Here's how the part is built. I have some questions about the finished solid (model axes, mm). Face numbers are marked on the shaded views. A direction names the side the tool comes from. Give positions to 0.01 mm unless a question says otherwise; leave off trailing zeros. Write each loop counter-clockwise with the first axis right and the second up, starting at its lowest first coordinate (ties: lowest second). Pieces come first, ordered by that corner, then holes. Notation, with made-up numbers: (64, -26) - (80, -26) arc R35 cw to (80, 6) - close; hole circle Ø10 at (6.25, 74.25). An arc over 180 degrees is marked (long way). One line per item, written item: value. Start each with the question number.
1) Imagine slicing it at C-C on x = -51.5. Write out the boundary of the cut face in (y, z) (3 decimals).
2) Imagine slicing it at B-B on y = 42. Write out the boundary of the cut face in (x, z) (3 decimals), plus the area to 3 significant figures.
3) I'm going to push flat-ended pins straight in: P1, Ø7.5, axis at y = -6, z = -5.5, coming from the -X side; P2, Ø4.5, axis at y = 8.5, z = 0, coming from the -X side; P3, Ø7, axis at x = 1, z = 7.5, coming from the +Y side; P4, Ø3.5, axis at x = -46.88, y = 72.87, coming from the -Z side. Where does each tip first touch, or does it pass through?
4) Imagine slicing it at A-A on z = 8.5. Write out the boundary of the cut face in (x, y) (3 decimals).
5) We'd pull the mould along Z, two halves only. Please class the marked faces 1, 2 and 3: +Z half, -Z half, draft (parallel to the pull), parting line (faces both ways), or undercut.
6) Imagine slicing it at D-D on y = 0. Count the separate pieces of the cut face and the enclosed holes in it, plus the area to 3 significant figures.
7) Please list where these lines run through material, in increasing order: L1, parallel to Y at x = 2.75, z = 0; L2, parallel to Z at x = 2, y = 0; L3, parallel to Z at x = -31, y = 48 (3 decimals). Write a range as [from, to].
8) On a 3-axis mill with a long thin cutter (end or side, diameter ignored), from which of +Z, -Z, +X, -X, +Y, -Y can I reach the whole of each face in a straight line? I mean the marked faces 4 and 5. Say none if no direction works.
from build123d import *

# Parameters (mm, degrees)
SKETCH2_W                                      = 29
SKETCH2_H                                      = 25
BOSS_EXTRUDE1_DEPTH                            = 6.35
CONVERT_SOLID1_START                           = 3.175
CONVERT_SOLID1_OUTLINE_W                       = 25
CONVERT_SOLID1_OUTLINE_H                       = 29
CONVERT_SOLID1_DEPTH                           = 3.175
CSK_FOR_M3_5_FLAT_HEAD_MACHINE_SCREW1_AT_COUNT = 2
CSK_FOR_M3_5_FLAT_HEAD_MACHINE_SCREW1_AT_PITCH = 12.02081528
CSK_FOR_M3_5_FLAT_HEAD_MACHINE_SCREW_2_COUNT   = 2
CSK_FOR_M3_5_FLAT_HEAD_MACHINE_SCREW_2_PITCH   = 17
CSK_FOR_M3_5_FLAT_HEAD_MACHINE_SCREW_3_COUNT   = 2
CSK_FOR_M3_5_FLAT_HEAD_MACHINE_SCREW_3_PITCH   = 12.02081528
EDGE_FLANGE1_DEPTH                             = 25
EDGE_FLANGE1_BEND_DEPTH                        = 25
SKETCH23_R                                     = 1.95
SKETCH23_R_2                                   = 6.875
BOSS_EXTRUDE2_DEPTH                            = 3.175
FILLET1_R                                      = 40
SKETCH25_R                                     = 1.95
SKETCH25_R_2                                   = 6.875
CUT_EXTRUDE3_DEPTH                             = 108.532674661
FILLET2_R                                      = 2


# Read off the part's stored shape, not the designer's step: Convert-Solid1
# Sheet-metal steps are written as plain solids
with BuildPart() as part:
    # Sketch2 → Boss-Extrude1 (new body)
    with BuildSketch(Plane(origin=(0, 0, 0), x_dir=(0, 0, -1), z_dir=(1, 0, 0))):
        Rectangle(SKETCH2_W, SKETCH2_H)
    extrude(amount=BOSS_EXTRUDE1_DEPTH)

    # Convert-Solid1 outline → Convert-Solid1 (cut)
    with BuildSketch(Plane.YZ.offset(CONVERT_SOLID1_START)):
        Rectangle(CONVERT_SOLID1_OUTLINE_W, CONVERT_SOLID1_OUTLINE_H)
    extrude(amount=CONVERT_SOLID1_DEPTH, mode=Mode.SUBTRACT)

    # Sketch4 → CSK for M3.5 Flat Head Machine Screw1 (revolve, cut)
    with BuildSketch(Plane.ZX.offset(-8.5)):
        Polygon((0, 0), (0, 3.175), (1.95, 3.175), (1.95, 2.15), (4.1, 0), align=None)
    csk_for_m3_5_flat_head_machine_screw1 = revolve(axis=Axis((-6.35, -8.5, 0), (1, 0, 0)), mode=Mode.SUBTRACT)

    # CSK for M3.5 Flat Head Machine Screw1 at: CSK for M3.5 Flat Head Machine Screw1 ×2
    with Locations(*[Vector(0, 0.7071067811865476, 0.7071067811865476) * (i * CSK_FOR_M3_5_FLAT_HEAD_MACHINE_SCREW1_AT_PITCH) for i in range(1, CSK_FOR_M3_5_FLAT_HEAD_MACHINE_SCREW1_AT_COUNT)]):
        add(csk_for_m3_5_flat_head_machine_screw1, mode=Mode.SUBTRACT)

    # CSK for M3.5 Flat Head Machine Screw 2: CSK for M3.5 Flat Head Machine Screw1 ×2
    with Locations(*[(0, i * CSK_FOR_M3_5_FLAT_HEAD_MACHINE_SCREW_2_PITCH, 0) for i in range(1, CSK_FOR_M3_5_FLAT_HEAD_MACHINE_SCREW_2_COUNT)]):
        add(csk_for_m3_5_flat_head_machine_screw1, mode=Mode.SUBTRACT)

    # CSK for M3.5 Flat Head Machine Screw 3: CSK for M3.5 Flat Head Machine Screw1 ×2
    with Locations(*[Vector(0, 0.7071067811865476, -0.7071067811865476) * (i * CSK_FOR_M3_5_FLAT_HEAD_MACHINE_SCREW_3_PITCH) for i in range(1, CSK_FOR_M3_5_FLAT_HEAD_MACHINE_SCREW_3_COUNT)]):
        add(csk_for_m3_5_flat_head_machine_screw1, mode=Mode.SUBTRACT)

    # Edge-Flange1 section (across the edge) → Edge-Flange1 (add)
    with BuildSketch(Plane(origin=(0, 12.5, -17.675), x_dir=(0, 0, 1), z_dir=(0, -1, 0))):
        with BuildLine():
            Line((-3.175, 3.175), (-3.175, 36.825))
            Line((-3.175, 36.825), (0, 36.825))
            Line((0, 36.825), (0, 3.175))
            ThreePointArc((0, 3.175), (0.92993597, 0.92993597), (3.175, 0))
            Line((3.175, 0), (3.175, -3.175))
            ThreePointArc((3.175, -3.175), (-1.315128061, -1.315128061), (-3.175, 3.175))
        make_face()
    extrude(amount=EDGE_FLANGE1_DEPTH)

    # Edge-Flange1 section 2 (across the edge) → Edge-Flange1 bend (add)
    with BuildSketch(Plane(origin=(0, -12.5, 17.675), x_dir=(0, 0, -1), z_dir=(0, 1, 0))):
        with BuildLine():
            Line((-3.175, 3.175), (-3.175, 36.825))
            Line((-3.175, 36.825), (0, 36.825))
            Line((0, 36.825), (0, 3.175))
            ThreePointArc((0, 3.175), (0.92993597, 0.92993597), (3.175, 0))
            Line((3.175, 0), (3.175, -3.175))
            ThreePointArc((3.175, -3.175), (-1.315128061, -1.315128061), (-3.175, 3.175))
        make_face()
    extrude(amount=EDGE_FLANGE1_BEND_DEPTH)

    # Sketch23 → Boss-Extrude2 (add)
    with BuildSketch(Plane.XY.offset(20.85)):
        with BuildLine():
            Line((-3.175, -12.5), (-3.175, 12.5))
            Line((-3.175, 12.5), (-39.000765285, 77.226355048))
            ThreePointArc((-39.000765285, 77.226355048), (-50.077531286, 81.278922457), (-55.654025191, 70.885618681))
            Line((-55.654025191, 70.885618681), (-36.825, -12.5))
            Line((-36.825, -12.5), (-3.175, -12.5))
        make_face()
        with Locations((-46.875056501, 72.867967978)):
            Circle(SKETCH23_R, mode=Mode.SUBTRACT)
        with Locations((-29.474943499, 27.168448642)):
            Circle(SKETCH23_R, mode=Mode.SUBTRACT)
        with Locations((-38.175, 50.01820831)):
            Circle(SKETCH23_R_2, mode=Mode.SUBTRACT)
    boss_extrude2 = extrude(amount=-BOSS_EXTRUDE2_DEPTH)

    # Mirror3: Boss-Extrude2 across plane
    add(boss_extrude2.mirror(Plane.XY))

    # Fillet1
    fillet1_edges = [part.edges().sort_by_distance(p)[0] for p in [
        (-36.825, -12.5, -19.2625),
        (-36.825, -12.5, 19.2625),
    ]]
    fillet(fillet1_edges, radius=FILLET1_R)

    # Sketch25 → Cut-Extrude3 (cut, through all)
    with BuildSketch(Plane.XY.offset(20.85)):
        with Locations((-46.875056501, 72.867967978)):
            Circle(SKETCH25_R)
        with Locations((-38.175, 50.01820831)):
            Circle(SKETCH25_R_2)
        with Locations((-29.474943499, 27.168448642)):
            Circle(SKETCH25_R)
        with BuildLine():
            Line((-40.192024973, 20.647751172), (-31.28455236, 22.659117506))
            Line((-31.28455236, 22.659117506), (-10.974113473, -7.975305792))
            ThreePointArc((-10.974113473, -7.975305792), (-30.042886429, 1.783719979), (-40.192024973, 20.647751172))
        make_face()
    extrude(amount=-CUT_EXTRUDE3_DEPTH, mode=Mode.SUBTRACT)

    # Fillet2
    fillet2_edges = [part.edges().sort_by_distance(p)[0] for p in [
        (-31.28455236, 22.659117506, 19.2625),
        (-10.974113473, -7.975305792, 19.2625),
        (-40.192024973, 20.647751172, 19.2625),
        (-31.28455236, 22.659117506, -19.2625),
        (-10.974113473, -7.975305792, -19.2625),
        (-40.192024973, 20.647751172, -19.2625),
    ]]
    fillet(fillet2_edges, radius=FILLET2_R)


solid = part.part
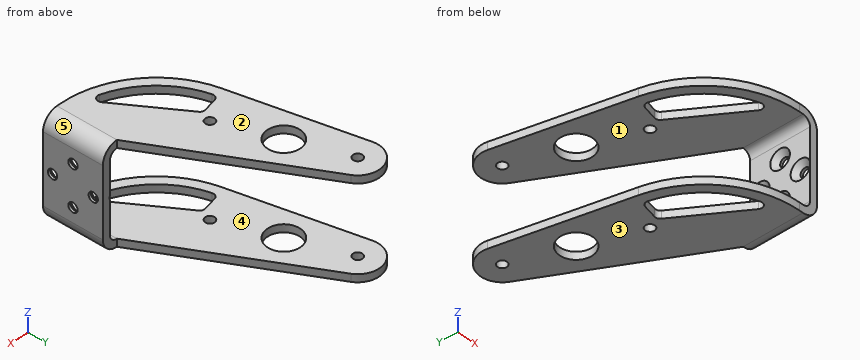
Numbers:
1. outline: (52.489, -20.85) - (80.589, -20.85) - (80.589, -17.675) - (52.489, -17.675) - close; (52.489, 17.675) - (80.589, 17.675) - (80.589, 20.85) - (52.489, 20.85) - close
2. outline: (-49.131, -20.85) - (-19.503, -20.85) - (-19.503, -17.675) - (-49.131, -17.675) - close; (-49.131, 17.675) - (-19.503, 17.675) - (-19.503, 20.85) - (-49.131, 20.85) - close
2. area: 188 mm^2
3. P1: x = 0
3. P2: x = 1.85
3. P3: y = 12.5
3. P4: through
4. outline: (0, -12.5) - (3.175, -12.5) - (3.175, -1.95) - (2.15, -1.95) - (0, -4.1) - close; (0, 4.1) - (2.15, 1.95) - (3.175, 1.95) - (3.175, 12.5) - (0, 12.5) - close
5. face 1: undercut
5. face 2: +Z half
5. face 3: -Z half
6. separate pieces: 5
6. enclosed holes: 0
6. area: 226 mm^2
7. L1: [-12.5, -10.45], [-6.55, 6.55], [10.45, 12.5]
7. L2: [-18.18, -10.6], [-6.4, 6.4], [10.6, 18.18]
7. L3: [-20.85, -17.675], [17.675, 20.85]
8. face 4: -X, +Y, -Y
8. face 5: +Z, +X, +Y, -Y
